Can you work these out from the drawing? Everything is in mm from the part's minimum corner. A direction names the side the tool comes from. Coordinates: 2 decimals unless noted, no trailing zeros. Loops run counter-clockwise (first coordinate to the right, second up) from the corner with the lowest first, then second, coordinate; pieces in that order, holes last.
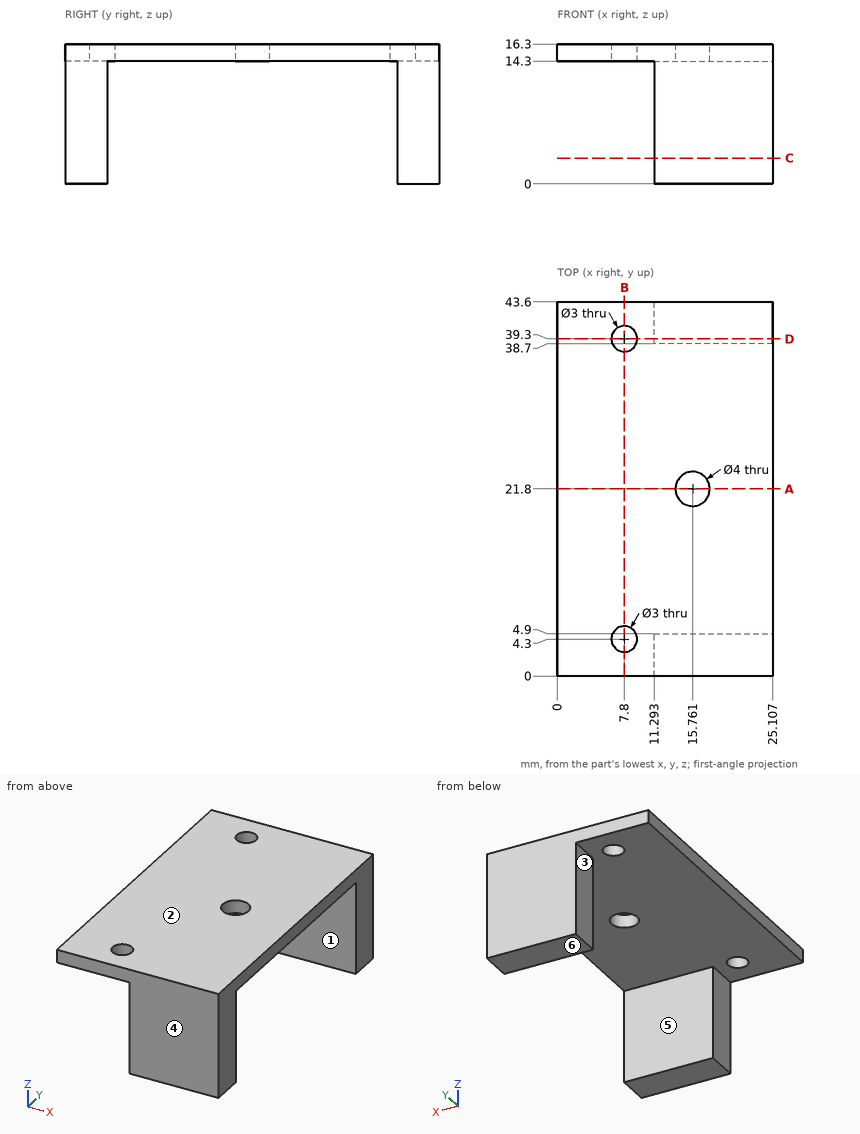
(1) I need wall thicknesses on probe 1 along Y at (x, z) = (7.8, 14.85); probe 2 along Y at (x, z) = (18.5, 10.25); probe 3 along Z at (x, y) = (3.5, 41.5). Which ranges of each line are inside material? Lowest first, please.
Answers:
probe 1: y = 0 to 2.8, 5.8 to 37.8, 40.8 to 43.6
probe 2: y = 0 to 4.9, 38.7 to 43.6
probe 3: z = 14.3 to 16.3
(2) For pin 1 (6.5 mm diameter, centred on x = 15.76, y = 21.8, fed in from +Z); pin 2 (2.5 mm diameter, centred on y = 1.5, z = 4, fed in from -X); pin 3 (12.5 mm diameter, centred on x = 17, y = 22, fed in from -Z); pin 4 (1.5 mm diameter, centred on y = 10.5, z = 13, fed in from -X), each with a flat end and sliding along its axis, tell me the tip position at first contact or that it passes through.
Answers:
pin 1: stops at z = 16.3
pin 2: stops at x = 11.29
pin 3: stops at z = 14.3
pin 4: passes through
(3) Imagine slicing it at D-D, the plane y = 39.3. Write out the boundary of the cut face in (x, z).
Answers:
outline: (0, 14.3) - (6.3, 14.3) - (6.3, 16.3) - (0, 16.3) - close; (9.3, 14.3) - (11.29, 14.3) - (11.29, 0) - (25.11, 0) - (25.11, 16.3) - (9.3, 16.3) - close
(4) Imagine slicing it at C-C, the plane z = 3. Write out the boundary of the cut face in (x, y), and give its area (3 significant figures).
Answers:
outline: (11.29, 0) - (25.11, 0) - (25.11, 4.9) - (11.29, 4.9) - close; (11.29, 38.7) - (25.11, 38.7) - (25.11, 43.6) - (11.29, 43.6) - close
area: 135 mm2
(5) Which directions (+Z, -Z, +X, -X, +Y, -Y) give clear straight access to the entire face, cutting with the end or side of a thin tool? Please do the marked faces 1, 2 and 3.
Answers:
face 1: -Z, +X, -X
face 2: +Z, +X, -X, +Y, -Y
face 3: -Z, -X, +Y, -Y
(6) Imagine slicing it at B-B, the plane x = 7.8. Write out the boundary of the cut face in (y, z).
Answers:
outline: (0, 14.3) - (2.8, 14.3) - (2.8, 16.3) - (0, 16.3) - close; (5.8, 14.3) - (37.8, 14.3) - (37.8, 16.3) - (5.8, 16.3) - close; (40.8, 14.3) - (43.6, 14.3) - (43.6, 16.3) - (40.8, 16.3) - close
(7) Imagine slicing it at A-A, the plane y = 21.8. Write out the boundary of the cut face in (x, z).
Answers:
outline: (0, 14.3) - (13.76, 14.3) - (13.76, 16.3) - (0, 16.3) - close; (17.76, 14.3) - (25.11, 14.3) - (25.11, 16.3) - (17.76, 16.3) - close
(8) We'd pull the mould along Y, two halves only. Please class the marked faces 4, 5 and 6: +Y half, -Y half, draft (parallel to the pull), parting line (faces both ways), or undercut.
Answers:
face 4: -Y half
face 5: undercut
face 6: draft
